Could you check a few things on this model? Use its own coordinates, in mm. A direction names the side the tool comes from. Coordinates: 2 decimals unless noted, no trailing zeros. Order: outer loops, then holes, each group sorted by start corner. A loop starts at its lowest first (then second) coordinate and runs counter-clockwise, first axis right, second up. Notation, with made-up numbers: (34.25, -21.5) - (57.25, -21.5) arc R28 ccw to (57.25, 10.5) - close; hole circle Ø2 at (59.5, -19). An arc over 180 degrees is marked (long way). Answer as a JSON object with one key per item and string values. Group by question number.
(1) Imagine slicing it at B-B, the plane x = -10.5. Write out the boundary of the cut face in (y, z), and give its area (4 significant figures).
(2) Imagine slicing it at D-D, the plane x = 4.25. Write out the boundary of the cut face in (y, z), and give its area (3 significant figures).
(3) Please list where these lines run through material, in increasing order: probe 1 along X at (y, z) = (0.3, -10.5); probe 2 along Y at (x, z) = (-11.5, 8.25); probe 3 along X at (y, z) = (2.5, -2.5).
(4) We'd pull the mould along Z, two halves only. Please class faces 1 (the flat face through (4, 2, 0)), 2 (the flat face through (-2, 6, 0)), 3 (the flat face through (-9, -1, -11.75)), 4 (the cylindrical face through (-3.1, 0.5, -11.3)): pulls with the +Z half, pulls with the -Z half, needs draft (parallel to the pull), parting line crosses it, or undercut.
(5) Imagine slicing it at C-C, the plane y = 1.5. Write out the boundary of the cut face in (x, z), and give its area (3 significant figures).
(6) Will these pins go through, and if not, where does the flat tip stop? P1, Ø2, axis at x = 6.5, y = 2.5, coming from the -Z side; P2, Ø3, axis at x = 10, z = -10.5, coming from the +Y side; P3, Ø1.5, axis at x = -14, z = 4, coming from the -Y side.
(7) Which directions (+Z, -Z, +X, -X, +Y, -Y) give clear straight access to the entire face, cutting with the end or side of a thin tool? Please do faces 5 (the flat face through (-3, 4, -4)), 6 (the flat face through (-13, -1.837, 0)).
from build123d import *

# Parameters (mm, degrees)
SKETCH_1_W          = 24
SKETCH_1_H          = 25
EXTRUDE_1_DEPTH     = 1
SKETCH_2_W          = 8.5
SKETCH_2_H          = 8.5
EXTRUDE_2_DEPTH     = 3
SKETCH_3_R          = 4
EXTRUDE_3_DEPTH     = 2
SKETCH_4_W          = 3
SKETCH_4_H          = 8.5
EXTRUDE_4_DEPTH     = 2
SKETCH_5_W          = 2.95
SKETCH_5_H          = 6.47612255
EXTRUDE_5_DEPTH     = 1
SKETCH_6_W          = 4
SKETCH_6_H          = 23.5
EXTRUDE_6_DEPTH     = 2.5
CHAMFER_1_SIZE      = 1
SKETCH_7_W          = 20.993550262
SKETCH_7_H          = 0.673046144
EXTRUDE_7_DEPTH     = 5
SKETCH_8_R          = 1
CUT_EXTRUDE_1_DEPTH = 1
SKETCH_9_R          = 3.5
EXTRUDE_8_DEPTH     = 0.2
SKETCH_10_R         = 0.75
CUT_EXTRUDE_2_DEPTH = 0.2


with BuildPart() as part:
    # 草图1 → 凸台-拉伸1 (new body)
    with BuildSketch(Plane(origin=(0, 0, 0), x_dir=(1, 0, 0), z_dir=(0, 1, 0))):
        Rectangle(SKETCH_1_W, SKETCH_1_H)
    extrude(amount=EXTRUDE_1_DEPTH)

    # 草图2 → 凸台-拉伸2 (add)
    with BuildSketch(Plane(origin=(0, 1, 0), x_dir=(1, 0, 0), z_dir=(0, 1, 0))):
        with Locations((-1.7, 0)):
            Rectangle(SKETCH_2_W, SKETCH_2_H)
    extrude(amount=EXTRUDE_2_DEPTH)

    # 草图3 → 凸台-拉伸3 (add)
    with BuildSketch(Plane(origin=(0, 4, 0), x_dir=(1, 0, 0), z_dir=(0, 1, 0))):
        with Locations(Location((-1.7, 0, 0), (0, 0, 270))):
            Circle(SKETCH_3_R)
    extrude(amount=EXTRUDE_3_DEPTH)

    # 草图4 → 凸台-拉伸4 (add)
    with BuildSketch(Plane(origin=(0, 1, 0), x_dir=(1, 0, 0), z_dir=(0, 1, 0))):
        with Locations((7, -0.004190874)):
            Rectangle(SKETCH_4_W, SKETCH_4_H)
    extrude(amount=EXTRUDE_4_DEPTH)

    # 草图5 → 凸台-拉伸5 (add)
    with BuildSketch(Plane(origin=(0, 1, 0), x_dir=(1, 0, 0), z_dir=(0, 1, 0))):
        with Locations((4.025, 0)):
            Rectangle(SKETCH_5_W, SKETCH_5_H)
    extrude(amount=EXTRUDE_5_DEPTH)

    # 草图6 → 凸台-拉伸6 (add)
    with BuildSketch(Plane(origin=(0, 0, 0), x_dir=(1, 0, 0), z_dir=(0, 1, 0))):
        with Locations((-9, 0)):
            Rectangle(SKETCH_6_W, SKETCH_6_H)
    extrude(amount=-EXTRUDE_6_DEPTH)

    # 倒角1
    chamfer_1_edges = [part.edges().sort_by_distance(p)[0] for p in [
        (-7, -2.5, 0),
    ]]
    chamfer(chamfer_1_edges, length=CHAMFER_1_SIZE)

    # 草图7 → 凸台-拉伸7 (add)
    with BuildSketch(Plane.ZY.offset(11)):
        with Locations((0, -1.5)):
            Rectangle(SKETCH_7_W, SKETCH_7_H)
    extrude(amount=EXTRUDE_7_DEPTH)

    # 草图8 → 切除-拉伸1 (cut)
    with BuildSketch(Plane(origin=(0, 1, 0), x_dir=(1, 0, 0), z_dir=(0, 1, 0))):
        with Locations(Location((10, -10.5, 0), (0, 0, 270))):
            Circle(SKETCH_8_R)
        with Locations(Location((10, 10.5, 0), (0, 0, 270))):
            Circle(SKETCH_8_R)
        with Locations(Location((-2.5, -10.5, 0), (0, 0, 270))):
            Circle(SKETCH_8_R)
        with Locations(Location((-2.5, 10.5, 0), (0, 0, 270))):
            Circle(SKETCH_8_R)
    extrude(amount=-CUT_EXTRUDE_1_DEPTH, mode=Mode.SUBTRACT)

    # 草图9 → 凸台-拉伸8 (add)
    with BuildSketch(Plane(origin=(0, 6, 0), x_dir=(1, 0, 0), z_dir=(0, 1, 0))):
        with Locations(Location((-1.7, 0, 0), (0, 0, 270))):
            Circle(SKETCH_9_R)
    extrude(amount=EXTRUDE_8_DEPTH)

    # 草图10 → 切除-拉伸2 (cut)
    with BuildSketch(Plane(origin=(0, 6.2, 0), x_dir=(1, 0, 0), z_dir=(0, 1, 0))):
        with Locations(Location((-1.7, 0, 0), (0, 0, 270))):
            Circle(SKETCH_10_R)
    extrude(amount=-CUT_EXTRUDE_2_DEPTH, mode=Mode.SUBTRACT)


solid = part.part
Result set:
{
 "1": {"outline": "(-2.5, -11.75) - (0, -11.75) - (0, -12.5) - (1, -12.5) - (1, 12.5) - (0, 12.5) - (0, 11.75) - (-2.5, 11.75) - close", "area": "83.75 mm^2"},
 "2": {"outline": "(0, -12.5) - (1, -12.5) - (1, -3.24) - (2, -3.24) - (2, 3.24) - (1, 3.24) - (1, 12.5) - (0, 12.5) - close", "area": "31.5 mm^2"},
 "3": {"probe 1": "x = -12 to -3.5, -1.5 to 9, 11 to 12", "probe 2": "y = -1.84 to -1.16, 0 to 1", "probe 3": "x = -5.95 to 2.55, 5.5 to 8.5"},
 "4": {"face 1": "needs draft", "face 2": "undercut", "face 3": "pulls with the -Z half", "face 4": "undercut"},
 "5": {"outline": "(-5.95, -4.25) - (2.55, -4.25) - (2.55, -3.24) - (5.5, -3.24) - (5.5, -4.25) - (8.5, -4.25) - (8.5, 4.25) - (5.5, 4.25) - (5.5, 3.24) - (2.55, 3.24) - (2.55, 4.25) - (-5.95, 4.25) - close", "area": "117 mm^2"},
 "6": {"P1": "stops at z = -4.25", "P2": "stops at y = 1", "P3": "stops at y = -1.84"},
 "7": {"face 5": "+Y", "face 6": "+Z, -Z, -X, -Y"}
}
